Input: dimensioned drawing with shaded views. Units: mm. Origin: part minimum x, y, z. A direction names the side the tool comes from. Round coordinates to 2 decimals unless told otherwise and drop trailing zeros. Write each loop counter-clockwise with the first axis right and the second up, starting at its lowest first coordinate (ties: lowest second). Pieces come first, ordered by that corner, then holes. Notation, with made-up numbers: (38, 82) -> (82, 82) arc R24 cw to (82, 103) -> close; hole circle Ø11 at (54.25, 49). An arc over 180 degrees is marked (long way). One line per item, written item: value. Start each with the question number.
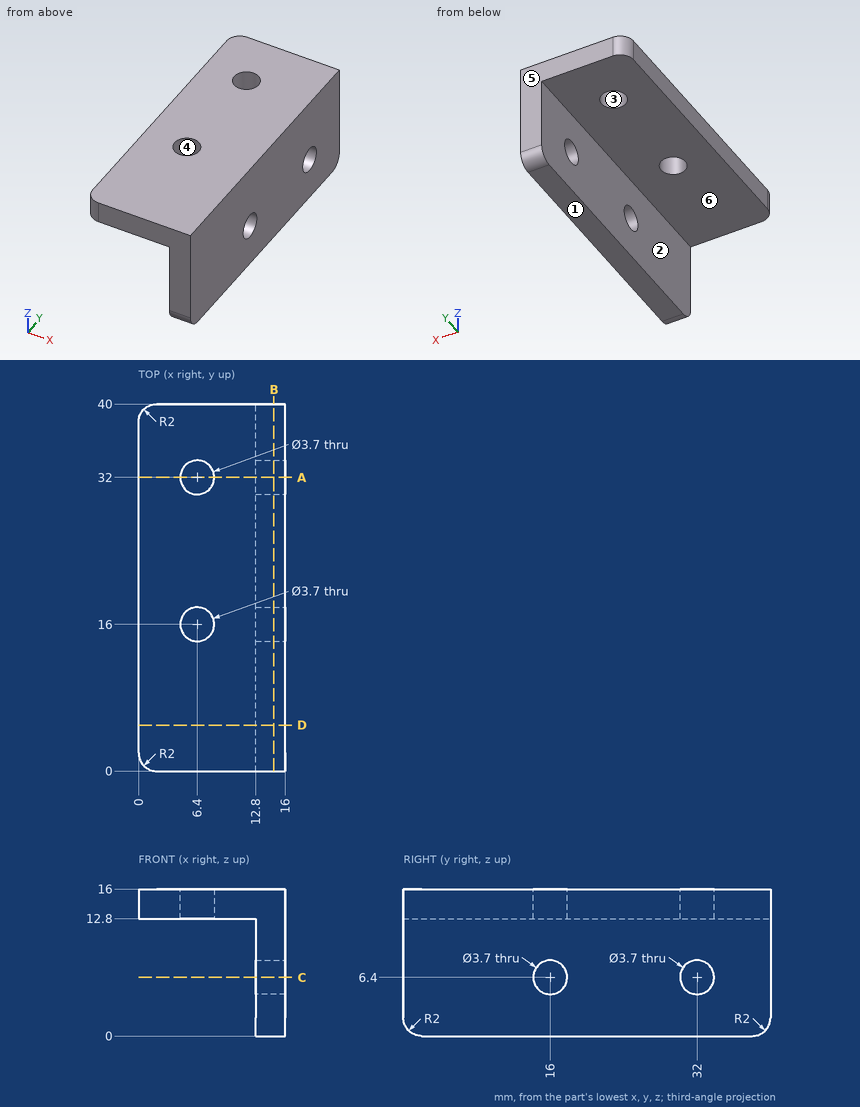
(1) Section query D-D (y = 5). Output: boundary loops of the cut face in (x, z).
(2) Section query A-A (y = 32). Output: boundary loops of the cut face in (x, z).
(3) Line query: probe 1 along Y at (x, z) = (6.4, 13.5); probe 2 along X at (y, z) = (19.5, 3.25). Output: solid intervals per line, ascending.
(4) Pull-direction query (Y, two-part tool) for the marked faces 3, 4, 5 and 6; classes: pulls with the +Y half, pulls with the -Y half, needs draft (parallel to the pull), parting line crosses it, or undercut.
(5) Section query C-C (z = 6.4). Output: boundary loops of the cut face in (x, y), and give its area (3 significant figures).
(6) Set-up query: the marked faces 1 and 2. Return all of +Z, -Z, +X, -X, +Y, -Y with unobstructed straight access to the full face (end or side cutting, diameter ignored); none if empty.
(7) Section query B-B (x = 14.75). Output: boundary loops of the cut face in (y, z).
(8) Pin query (flat end, axial travel): pin 1 (6 mm diameter, centred on x = 6.4, y = 32, fed in from -Z); pin 2 (6.5 mm diameter, centred on y = 25, z = 3.5, fed in from -X); pin 3 (2 mm diameter, centred on y = 16, z = 6.4, fed in from +X). Return the tip coordinate at first contact, or that it passes through.
Results list:
1. outline: (0, 12.8) -> (12.8, 12.8) -> (12.8, 0) -> (16, 0) -> (16, 16) -> (0, 16) -> close
2. outline: (0, 12.8) -> (4.55, 12.8) -> (4.55, 16) -> (0, 16) -> close; (8.25, 12.8) -> (12.8, 12.8) -> (12.8, 8.25) -> (16, 8.25) -> (16, 16) -> (8.25, 16) -> close; (12.8, 0) -> (16, 0) -> (16, 4.55) -> (12.8, 4.55) -> close
3. probe 1: y = 0 to 14.15, 17.85 to 30.15, 33.85 to 40
3. probe 2: x = 12.8 to 16
4. face 3: undercut
4. face 4: undercut
4. face 5: pulls with the +Y half
4. face 6: needs draft
5. outline: (12.8, 0) -> (16, 0) -> (16, 14.15) -> (12.8, 14.15) -> close; (12.8, 17.85) -> (16, 17.85) -> (16, 30.15) -> (12.8, 30.15) -> close; (12.8, 33.85) -> (16, 33.85) -> (16, 40) -> (12.8, 40) -> close
5. area: 104 mm^2
6. face 1: -Z, +X, -X, +Y, -Y
6. face 2: -Z, -X, +Y, -Y
7. outline: (0, 2) arc R2 ccw to (2, 0) -> (38, 0) arc R2 ccw to (40, 2) -> (40, 16) -> (0, 16) -> close; hole circle Ø3.7 at (16, 6.4); hole circle Ø3.7 at (32, 6.4)
8. pin 1: stops at z = 12.8
8. pin 2: stops at x = 12.8
8. pin 3: passes through
